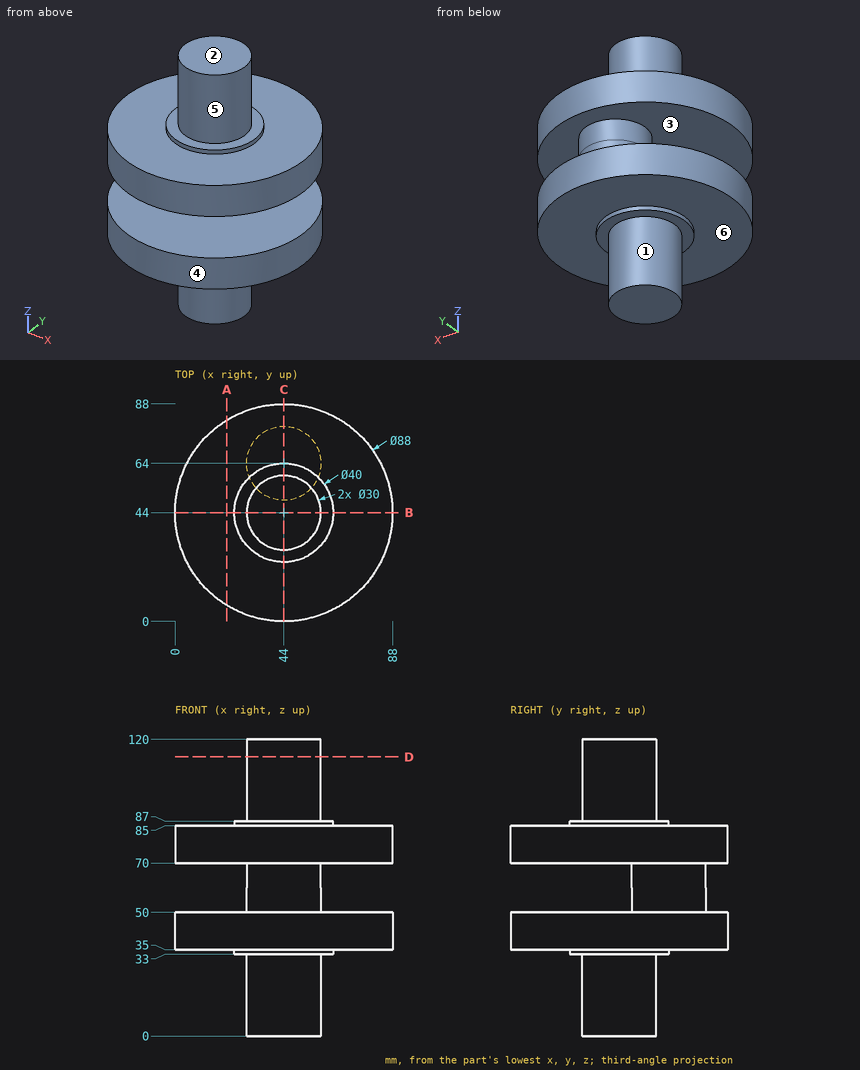
The drawing under review shows one solid part. Ordinate dimensions are in mm from its lowest x, y, z. A direction names the side the tool comes from. Round coordinates to 2 decimals unless told otherwise and drop trailing zeros. Loops run counter-clockwise (first coordinate to the right, second up) from the corner with the lowest first, then second, coordinate; pieces in that order, holes last. Notation, with made-up numbers: (25, 87.25) -> (78, 87.25) arc R22 ccw to (78, 113.25) -> close; hole circle Ø3 at (78.25, -11). An arc over 180 degrees is marked (long way). One line per question, with ' | ' between items. Start each with the question number.
Item 1: For pin 1 (1 mm diameter, centred on x = 26, y = 10.5, fed in from +Z); pin 2 (2 mm diameter, centred on y = 25, z = 38.5, fed in from -X); pin 3 (6 mm diameter, centred on x = 53.5, z = 41.5, fed in from -Y), all flat-tipped, find the tip position at first contact; note any pin that passes through.
Item 2: Draft analysis for pull direction Z (two halves, no side actions). For the marked faces 1, 2 and 3, state which applies: +Z half, -Z half, draft (parallel to the pull), parting line (faces both ways), or undercut.
Item 3: Add section C-C, the plane x = 44. Write out the cut boundary in (y, z), then the cut area to 3 significant figures.
Item 4: Machinability: for the marked faces 4, 5 and 6, which of the approach directions +Z, -Z, +X, -X, +Y, -Y give a long, thin tool a straight path to every point of the face, cutting with its end or side? Answer none if there is none.
Item 5: Add section D-D, the plane z = 113. Write out the cut boundary in (x, y).
Item 6: Add section A-A, the plane x = 21. Write out the cut boundary in (y, z).
Item 7: Add section B-B, the plane y = 44. Write out the cut boundary in (x, z), then the cut area to 3 significant figures.
Item 8: Wall thickness on line 1 along Z through (x, y) = (25.5, 68); line 2 along Z through (x, y) = (33, 32.5); line 3 along Z through (x, y) = (30, 67): over which ranges is each line inside the solid? List them lowest first. Write a range as [from, to].
Return value:
1) pin 1: stops at z = 85 | pin 2: stops at x = 3.85 | pin 3: stops at y = 0.48
2) face 1: draft | face 2: +Z half | face 3: undercut
3) outline: (0, 35) -> (24, 35) -> (24, 33) -> (29, 33) -> (29, 0) -> (59, 0) -> (59, 33) -> (64, 33) -> (64, 35) -> (88, 35) -> (88, 50) -> (79, 50) -> (79, 70) -> (88, 70) -> (88, 85) -> (64, 85) -> (64, 87) -> (59, 87) -> (59, 120) -> (29, 120) -> (29, 87) -> (24, 87) -> (24, 85) -> (0, 85) -> (0, 70) -> (49, 70) -> (49, 50) -> (0, 50) -> close | area: 5,380 mm2
4) face 4: +Z, -Z | face 5: +Z | face 6: -Z
5) outline: circle Ø30 at (44, 44)
6) outline: (6.49, 35) -> (81.51, 35) -> (81.51, 50) -> (6.49, 50) -> close; (6.49, 70) -> (81.51, 70) -> (81.51, 85) -> (6.49, 85) -> close
7) outline: (0, 35) -> (24, 35) -> (24, 33) -> (29, 33) -> (29, 0) -> (59, 0) -> (59, 33) -> (64, 33) -> (64, 35) -> (88, 35) -> (88, 50) -> (0, 50) -> close; (0, 70) -> (88, 70) -> (88, 85) -> (64, 85) -> (64, 87) -> (59, 87) -> (59, 120) -> (29, 120) -> (29, 87) -> (24, 87) -> (24, 85) -> (0, 85) -> close | area: 4,780 mm2
8) line 1: z = [35, 50], [70, 85] | line 2: z = [33, 50], [70, 87] | line 3: z = [35, 85]
